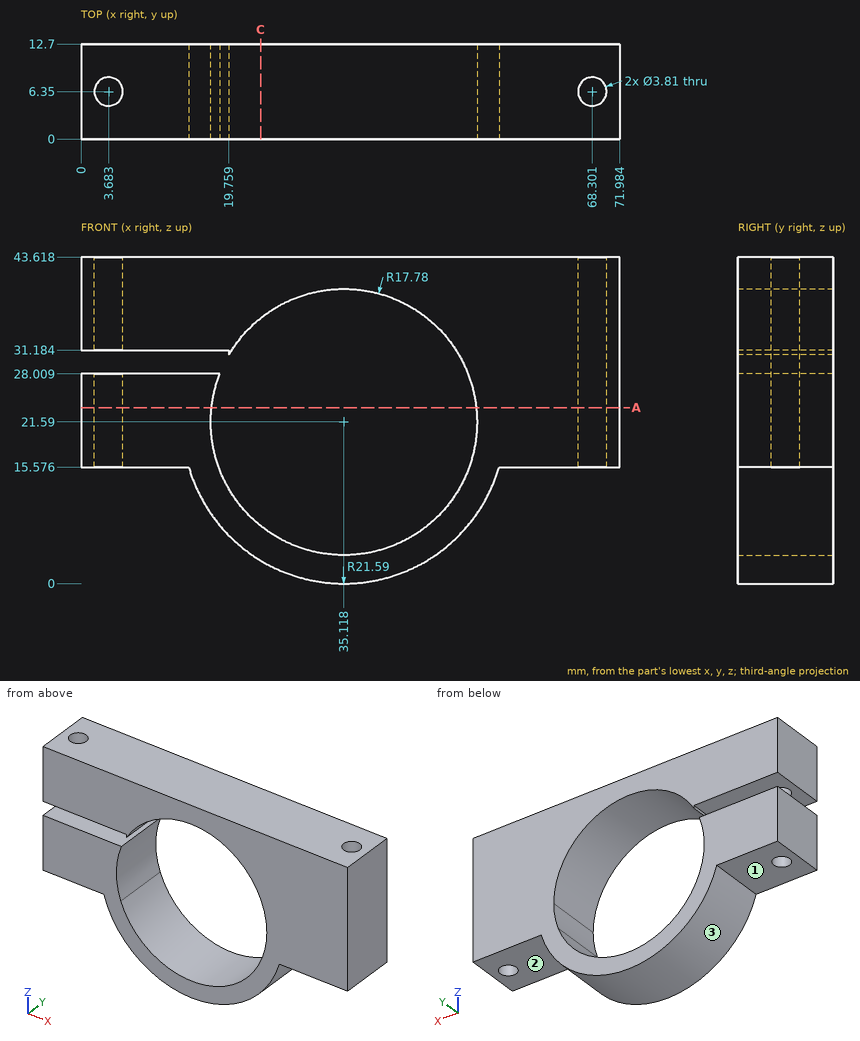
Print and shaded views of the part. All mm, measured from the part's lowest x, y and z. A direction names the side the tool comes from. Coordinates: 2 decimals unless noted, no trailing zeros. Order: outer loops, then holes, each group sorted by start corner. A loop starts at its lowest first (then second) coordinate and runs counter-clockwise, first axis right, second up. Notation, with made-up numbers: M 82,65.25 L 107,65.25 A25 cw 107,96.25 Z; hole C -26.75,18 d6. An arc over 180 degrees is marked long. One line per question, with ' | ' between items. Start each with the question number.
Q1. Flat gauge pins, fed straight in: pin 1 Ø4 at (x, y) = (6.5, 6) entering from -Z; pin 2 Ø8 at (x, z) = (27, 6.5) entering from +Y; pin 3 Ø3 at (x, y) = (3.683, 6.35) entering from -Z. Where does each tip first touch, or does it go through?
Q2. 3-axis set-ups, long thin cutter, end or side, ignore diameter. For the marked faces 1, 2 and 3: which of +Z, -Z, +X, -X, +Y, -Y reach the whole face in a straight line?
Q3. Saw through at A-A (z = 23.5). Count the separate pieces of the cut face and the enclosed holes in it.
Q4. Saw through at C-C (x = 24). List the corners of the cut face in (y, z) (1 decimal), then the cut area to 3 significant figures.
Q5. Probe L1, parallel to Y at x = 68.5, z = 38.5 (1 decimal); L2, parallel to Z at x = 58.5, y = 10; L3, parallel to Z at x = 5.5, y = 1 (1 decimal). List the from-to ranges inside material, lowest first. Write a range as from..to.
Check values:
1) pin 1: stops at z = 15.58 | pin 2: stops at y = 12.7 | pin 3: passes through
2) face 1: -Z, -X, +Y, -Y | face 2: -Z, +X, +Y, -Y | face 3: -Z, +Y, -Y
3) separate pieces: 2 | enclosed holes: 2
4) outline: M 0,3.1 L 12.7,3.1 L 12.7,7.7 L 0,7.7 Z; M 0,35.5 L 12.7,35.5 L 12.7,43.6 L 0,43.6 Z | area: 162 mm2
5) L1: y = 0..4.5, 8.2..12.7 | L2: z = 15.58..43.62 | L3: z = 15.6..28, 31.2..43.6
